from build123d import *

# Parameters (mm, degrees)
F0_R     = 3.175
F1_DEPTH = 4.7625
F2_R     = 6.35
F3_DEPTH = 4.7625


with BuildPart() as f1:
    # F0 (on Top) → F1 (new body)
    with BuildSketch(Plane.XY):
        with BuildLine():
            Line((10.4775, 13.335), (-10.4775, 13.335))
            ThreePointArc((-10.4775, 13.335), (-10.942468, 12.212468), (-12.065, 11.7475))
            Line((-12.065, 11.7475), (-12.065, -11.7475))
            ThreePointArc((-12.065, -11.7475), (-10.942468, -12.212468), (-10.4775, -13.335))
            Line((-10.4775, -13.335), (10.4775, -13.335))
            ThreePointArc((10.4775, -13.335), (10.942468, -12.212468), (12.065, -11.7475))
            Line((12.065, -11.7475), (12.065, 11.7475))
            ThreePointArc((12.065, 11.7475), (10.942468, 12.212468), (10.4775, 13.335))
        make_face()
        Circle(F0_R, mode=Mode.SUBTRACT)
    extrude(amount=F1_DEPTH)

    # F2 (on face) → F3 (join)
    with BuildSketch(Plane(origin=(0, 0, 0), x_dir=(1, 0, 0), z_dir=(0, 0, -1))):
        with BuildLine():
            ThreePointArc((10.4775, -13.335), (10.942468, -12.212468), (12.065, -11.7475))
            Line((12.065, -11.7475), (12.065, 11.7475))
            ThreePointArc((12.065, 11.7475), (10.942468, 12.212468), (10.4775, 13.335))
            Line((10.4775, 13.335), (-10.4775, 13.335))
            ThreePointArc((-10.4775, 13.335), (-10.942468, 12.212468), (-12.065, 11.7475))
            Line((-12.065, 11.7475), (-12.065, -11.7475))
            ThreePointArc((-12.065, -11.7475), (-10.942468, -12.212468), (-10.4775, -13.335))
            Line((-10.4775, -13.335), (10.4775, -13.335))
        make_face()
        Circle(F2_R, mode=Mode.SUBTRACT)
    extrude(amount=F3_DEPTH)


solid = f1.part
Input: part model. Units: mm. Frame: model coordinates. A direction names the side the tool comes from. Round coordinates to 2 decimals unless told otherwise and drop trailing zeros. Answer as CSV lines item,"result". Start each with the question number.
(1) Draft query along X for faces 1 (the cylindrical face through (-1.38, 6.2, -2.35)), 2 (the cylindrical face through (10.955, -12.2, 0.067)), 3 (the flat face through (0, 13.335, 0)). Return one class per face: released by +X, released by -X, zero draft, split by the parting line, or undercut.
(2) Reachability of faces 4 (the flat face through (-2, 3, 0)), 5 (the cylindrical face through (-10.93, -12.225, 0.067)) from +Z, -Z, +X, -X, +Y, -Y: full face, straight path, thin tool, end or side. Return the list, or none.
(3) First-contact query: pin 1 (10 mm diameter, centred on x = 0, y = 0, fed in from -Z). Flat tip, straight axial feed; report the tip coordinate or a pass-through.
(4) Line query: line 1 (X direction, y = 0, z = -3.1) (3 decimals); line 2 (Y direction, x = 0, z = -3.35) (3 decimals); line 3 (Y direction, x = 0, z = 2.2) (3 decimals). Output: solid intervals per line, ascending. Write a range as [from, to].
Values found:
1,face 1,"undercut"
1,face 2,"released by +X"
1,face 3,"zero draft"
2,face 4,"-Z"
2,face 5,"+Z, -Z, -X, -Y"
3,pin 1,"stops at z = 0"
4,line 1,"x = [-12.065, -6.35], [6.35, 12.065]"
4,line 2,"y = [-13.335, -6.35], [6.35, 13.335]"
4,line 3,"y = [-13.335, -3.175], [3.175, 13.335]"
